Read the model definition and answer for the solid it produces. Units are mm, in the model's axes. Give positions to 0.01 mm unless a question says otherwise; leave off trailing zeros. Order: outer loops, then holes, each group sorted by start corner. A loop starts at its lowest first (then second) coordinate and runs counter-clockwise, first axis right, second up. Notation, with made-up numbers: (16, 40) - (60, 40) arc R18 cw to (60, 69) - close; hole circle Ø1 at (32.25, 62). An arc over 180 degrees is marked (long way). Answer as CSV lines item,"result". Start each with the question number.
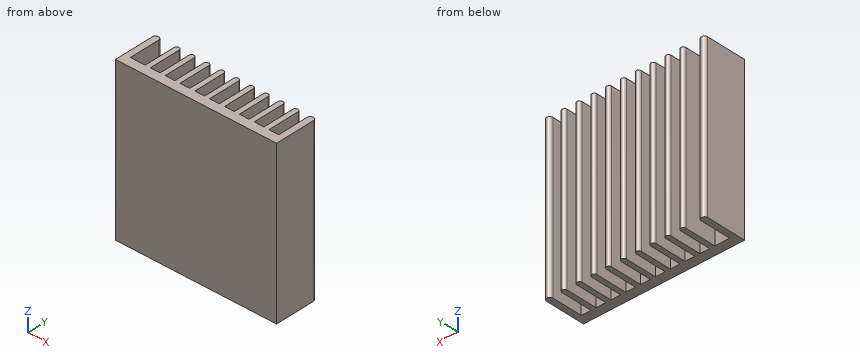
from build123d import *

# Parameters (mm, degrees)
EXTRUDE1_DEPTH = 38


with BuildPart() as part:
    # Sketch1 → Extrude1 (new body)
    with BuildSketch(Plane.XY):
        with BuildLine():
            Line((-19, 0), (19, 0))
            Line((19, 0), (19, 2.2))
            Line((19, 2.2), (19, 9.45))
            ThreePointArc((19, 9.45), (18.25, 10.2), (17.5, 9.45))
            Line((17.5, 9.45), (17.5, 2.2))
            Line((17.5, 2.2), (15.2, 2.2))
            Line((15.2, 2.2), (15.2, 9.6))
            ThreePointArc((15.2, 9.6), (14.6, 10.2), (14, 9.6))
            Line((14, 9.6), (14, 2.2))
            Line((14, 2.2), (11.7, 2.2))
            Line((11.7, 2.2), (11.7, 9.6))
            ThreePointArc((11.7, 9.6), (11.1, 10.2), (10.5, 9.6))
            Line((10.5, 9.6), (10.5, 2.2))
            Line((10.5, 2.2), (8.2, 2.2))
            Line((8.2, 2.2), (8.2, 9.6))
            ThreePointArc((8.2, 9.6), (7.6, 10.2), (7, 9.6))
            Line((7, 9.6), (7, 2.2))
            Line((7, 2.2), (4.7, 2.2))
            Line((4.7, 2.2), (4.7, 9.6))
            ThreePointArc((4.7, 9.6), (4.1, 10.2), (3.5, 9.6))
            Line((3.5, 9.6), (3.5, 2.2))
            Line((3.5, 2.2), (1.2, 2.2))
            Line((1.2, 2.2), (1.2, 9.6))
            ThreePointArc((1.2, 9.6), (0.6, 10.2), (0, 9.6))
            Line((0, 9.6), (0, 2.2))
            Line((0, 2.2), (-2.3, 2.2))
            Line((-2.3, 2.2), (-2.3, 9.6))
            ThreePointArc((-2.3, 9.6), (-2.9, 10.2), (-3.5, 9.6))
            Line((-3.5, 9.6), (-3.5, 2.2))
            Line((-3.5, 2.2), (-5.8, 2.2))
            Line((-5.8, 2.2), (-5.8, 9.6))
            ThreePointArc((-5.8, 9.6), (-6.4, 10.2), (-7, 9.6))
            Line((-7, 9.6), (-7, 2.2))
            Line((-7, 2.2), (-9.3, 2.2))
            Line((-9.3, 2.2), (-9.3, 9.6))
            ThreePointArc((-9.3, 9.6), (-9.9, 10.2), (-10.5, 9.6))
            Line((-10.5, 9.6), (-10.5, 2.2))
            Line((-10.5, 2.2), (-12.8, 2.2))
            Line((-12.8, 2.2), (-12.8, 9.6))
            ThreePointArc((-12.8, 9.6), (-13.4, 10.2), (-14, 9.6))
            Line((-14, 9.6), (-14, 2.2))
            Line((-14, 2.2), (-17.5, 2.2))
            Line((-17.5, 2.2), (-17.5, 9.45))
            ThreePointArc((-17.5, 9.45), (-18.25, 10.2), (-19, 9.45))
            Line((-19, 9.45), (-19, 2.2))
            Line((-19, 2.2), (-19, 0))
        make_face()
    extrude(amount=EXTRUDE1_DEPTH)


solid = part.part
(1) Section B-B, the plane x = 12.5 is taken. Write down the section's boundary in (y, z).
(2) Straight lines are drawn through the part: line 1 (Y direction, x = -4, z = 15.5); line 2 (Y direction, x = -2.5, z = 9.5). For each, find the intervals that lie inside material, in ascending order. Write a range as [from, to].
(3) Flat-ended cylindrical pins translate along their axes: pin 1 Ø1.5 at (x, z) = (6.5, 18) entering from +Y; pin 2 Ø1.2 at (x, z) = (-11.5, 18.5) entering from +Y. Find the tip coordinate at first contact, or state that the pin passes through.
(4) Section A-A, the plane y = 3.5 is taken. State how many separate pieces and enclosed holes the cut face has, and give its area (3 significant figures).
Checks:
1,outline,"(0, 0) - (2.2, 0) - (2.2, 38) - (0, 38) - close"
2,line 1,"y = [0, 2.2]"
2,line 2,"y = [0, 10.05]"
3,pin 1,"stops at y = 10.09"
3,pin 2,"stops at y = 2.2"
4,separate pieces,"11"
4,enclosed holes,"0"
4,area,"524 mm²"
